Work out the finished part from the listing and answer in its coordinate system (mm). A direction names the side the tool comes from. Coordinates: 2 decimals unless noted, no trailing zeros. Loops run counter-clockwise (first coordinate to the right, second up) from the corner with the lowest first, then second, coordinate; pieces in that order, holes last. Notation, with made-up numbers: (-38, 40.25) -> (-17, 40.25) arc R22 ccw to (-17, 72.25) -> close; hole circle Ø10 at (-26.5, -20). An arc over 180 degrees is marked (long way). Answer as CSV lines item,"result".
```python
from build123d import *

# Parameters (mm, degrees)
SKETCH1_W                = 20.2
SKETCH1_H                = 29
SKETCH1_W_2              = 16.2
SKETCH1_H_2              = 25
BOSS_EXTRUDE1_DEPTH      = 18.75
BOSS_EXTRUDE2_DEPTH      = 3.5
BOSS_EXTRUDE2_DEPTH_BACK = 2
SKETCH2_R                = 4.75
SKETCH3_W                = 43.2
SKETCH3_H                = 52
SKETCH3_W_2              = 16.2
SKETCH3_H_2              = 25
BOSS_EXTRUDE4_DEPTH      = 3.5


with BuildPart() as part:
    # Sketch1 → Boss-Extrude1 (new, symmetric)
    with BuildSketch(Plane(origin=(0, 0, 0), x_dir=(0, 0, -1), z_dir=(1, 0, 0))):
        Rectangle(SKETCH1_W, SKETCH1_H)
        Rectangle(SKETCH1_W_2, SKETCH1_H_2, mode=Mode.SUBTRACT)
    extrude(amount=BOSS_EXTRUDE1_DEPTH, both=True)

    # Sketch2 → Boss-Extrude2 (add, two sides: drawn at the far end of the back side and taken through both)
    with BuildSketch(Plane(origin=(0, 14.5, 0), x_dir=(1, 0, 0), z_dir=(0, 1, 0)).offset(-BOSS_EXTRUDE2_DEPTH_BACK)):
        with BuildLine():
            Line((-18.75, -10.1), (-18.75, 10.1))
            Line((-18.75, 10.1), (-27.403040645, 7.346959355))
            ThreePointArc((-27.403040645, 7.346959355), (-34.75, 0), (-27.403040645, -7.346959355))
            Line((-27.403040645, -7.346959355), (-18.75, -10.1))
        make_face()
        with Locations(Location((-27.403040645, 0, 0), (0, 0, 270))):
            Circle(SKETCH2_R, mode=Mode.SUBTRACT)
    extrude(amount=BOSS_EXTRUDE2_DEPTH + BOSS_EXTRUDE2_DEPTH_BACK)

    # Sketch3 → Boss-Extrude4 (add)
    with BuildSketch(Plane(origin=(18.75, 0, 0), x_dir=(0, 0, -1), z_dir=(1, 0, 0))):
        Rectangle(SKETCH3_W, SKETCH3_H)
        Rectangle(SKETCH3_W_2, SKETCH3_H_2, mode=Mode.SUBTRACT)
    boss_extrude4 = extrude(amount=-BOSS_EXTRUDE4_DEPTH)

    # Mirror1: Boss-Extrude4 across plane
    add(boss_extrude4.mirror(Plane(origin=(0, 0, 0), x_dir=(0, 0, 1), z_dir=(1, 0, 0))))


solid = part.part
```
(1) For a pull along X with two mould halves and no side action, classify faces 4 (the face through (15.25, 0, 15)), 5 (the face through (-23.02, 15.21, -8.74)), 6 (the face through (-15.25, 0, 15)), 7 (the face through (-17, 26, 0)) as pulls with the +X half, pulls with the -X half, needs draft (parallel to the pull), parting line crosses it, or undercut.
Computed values:
face 4,"undercut"
face 5,"pulls with the -X half"
face 6,"undercut"
face 7,"needs draft"
(2) Flat-ended cylindrical pins translate along their axes: pin 1 Ø6 at (x, z) = (4, 4.5) entering from -Y; pin 2 Ø12 at (x, z) = (6, 9.5) entering from +Y; pin 3 Ø17.5 at (x, z) = (-29, 3.5) entering from +Y; pin 4 Ø10 at (y, z) = (2.5, -2) entering from +X. Find the tip coordinate at first contact, or state that the pin passes through.
Computed values:
pin 1,"y = -14.5"
pin 2,"y = 14.5"
pin 3,"y = 18"
pin 4,"through"
(3) Which of the six approach directions +Z, -Z, +X, -X, +Y, -Y give full straight-line access (tool end or side, diameter ignored) to faces 1 (the face through (-22, 18, 0)), 2 (the face through (0, 0, 8.1)), 3 (the face through (0, 0, 10.1))?
Computed values:
face 1,"+Z, -Z, -X, +Y"
face 2,"+X, -X"
face 3,"+Z, +Y, -Y"
(4) Consider line 1 along X through (y, z) = (16.4, 0); line 2 along Z through (x, y) = (7, 9); line 3 along Z through (x, y) = (-17.5, -2). Determine where each line is inside the solid, lowest interval first.
Computed values:
line 1,"-34.75 to -32.15, -22.65 to -15.25, 15.25 to 18.75"
line 2,"-10.1 to -8.1, 8.1 to 10.1"
line 3,"-21.6 to -8.1, 8.1 to 21.6"
(5) A cutting plane is placed at D-D, the plane z = 15. Write down the section's boundary in (x, y), and give its area (3 significant figures).
Computed values:
outline,"(-18.75, -26) -> (-15.25, -26) -> (-15.25, 26) -> (-18.75, 26) -> close; (15.25, -26) -> (18.75, -26) -> (18.75, 26) -> (15.25, 26) -> close"
area,"364 mm2"
(6) A cutting plane is placed at B-B, the plane z = 0. Write down the section's boundary in (x, y), and give its area (3 significant figures).
Computed values:
outline,"(-34.75, 12.5) -> (-32.15, 12.5) -> (-32.15, 18) -> (-34.75, 18) -> close; (-22.65, 12.5) -> (18.75, 12.5) -> (18.75, 26) -> (15.25, 26) -> (15.25, 14.5) -> (-15.25, 14.5) -> (-15.25, 26) -> (-18.75, 26) -> (-18.75, 18) -> (-22.65, 18) -> close; (-18.75, -26) -> (-15.25, -26) -> (-15.25, -14.5) -> (15.25, -14.5) -> (15.25, -26) -> (18.75, -26) -> (18.75, -12.5) -> (-18.75, -12.5) -> close"
area,"347 mm2"
(7) A cutting plane is placed at A-A, the plane x = 9. Write down the section's boundary in (y, z).
Computed values:
outline,"(-14.5, -10.1) -> (14.5, -10.1) -> (14.5, 10.1) -> (-14.5, 10.1) -> close; hole (-12.5, -8.1) -> (12.5, -8.1) -> (12.5, 8.1) -> (-12.5, 8.1) -> close"
(8) A cutting plane is placed at C-C, the plane y = 1.5. Write down the section's boundary in (x, z).
Computed values:
outline,"(-18.75, -21.6) -> (-15.25, -21.6) -> (-15.25, -10.1) -> (15.25, -10.1) -> (15.25, -21.6) -> (18.75, -21.6) -> (18.75, -8.1) -> (-18.75, -8.1) -> close; (-18.75, 8.1) -> (18.75, 8.1) -> (18.75, 21.6) -> (15.25, 21.6) -> (15.25, 10.1) -> (-15.25, 10.1) -> (-15.25, 21.6) -> (-18.75, 21.6) -> close"
